Input: part model. Units: mm. Frame: model coordinates. A direction names the side the tool comes from. Give positions to 0.01 mm unless a question says otherwise; leave off trailing zeros. Order: outer loops, then holes, each group sorted by start corner. A loop starts at its lowest first (then second) coordinate and runs counter-clockwise, first axis right, second up.
```python
from build123d import *

# Parameters (mm, degrees)
F0_W     = 41.91
F0_H     = 2.54
F1_DEPTH = 15.24
F0_H_2   = 24.13
F2_DEPTH = 2.54


with BuildPart() as f1:
    # F0 (on Front) → F1 (new body)
    with BuildSketch(Plane.XZ):
        with Locations((20.955, 25.4)):
            Rectangle(F0_W, F0_H)
        Polygon((41.91, 24.13), (41.91, 0), (41.91, -2.54), (44.45, -2.54), (44.45, 26.67), (41.91, 26.67), align=None)
        with Locations((20.955, -1.27)):
            Rectangle(F0_W, F0_H)
    extrude(amount=F1_DEPTH)

    # F0 (on Front) → F2 (join)
    with BuildSketch(Plane.XZ):
        with Locations((20.955, 12.065)):
            Rectangle(F0_W, F0_H_2)
    extrude(amount=F2_DEPTH)


solid = f1.part
```
1) Reachability of faces 5 (the face through (21, -2.54, 12)), 6 (the face through (25, -15.24, -1)) from +Z, -Z, +X, -X, +Y, -Y: full face, straight path, thin tool, end or side. Return the list, or none.
2) Cut plane A-A (y = -8.5). Return the cut outline in (x, z), then the cut area to 3 significant figures.
3) Line query: probe 1 along Z at (x, y) = (41.5, -7.5); probe 2 along X at (y, z) = (-9, 16.5); probe 3 along Y at (x, z) = (27.5, 11). Output: solid intervals per line, ascending.
4) Cut plane B-B (x = 39). Return the cut outline in (y, z).
5) Pull-direction query (Z, two-part tool) for faces 1 (the face through (23, -8, 26.67)), 2 (the face through (41.91, -9, 12)), 3 (the face through (21, -9, 24.13)), 4 (the face through (44.45, -8, 12)); classes: pulls with the +Z half, pulls with the -Z half, needs draft (parallel to the pull), parting line crosses it, or undercut.
6) First-contact query: P1, Ø10, axis at x = 15, z = 13.5, coming from the -Y side; P2, Ø4, axis at y = -11, z = 17, coming from the -X side. Flat tips, straight axial feed; report the tip coordinate or a pass-through.
7) Cut plane C-C (z = 19.75). Return the cut outline in (x, y), then the cut area to 3 significant figures.
Geometry says:
1. face 5: -X, -Y
1. face 6: +Z, -Z, +X, -X, -Y
2. outline: (0, -2.54) - (44.45, -2.54) - (44.45, 26.67) - (0, 26.67) - (0, 24.13) - (41.91, 24.13) - (41.91, 0) - (0, 0) - close
2. area: 287 mm2
3. probe 1: z = -2.54 to 0, 24.13 to 26.67
3. probe 2: x = 41.91 to 44.45
3. probe 3: y = -2.54 to 0
4. outline: (-15.24, -2.54) - (0, -2.54) - (0, 26.67) - (-15.24, 26.67) - (-15.24, 24.13) - (-2.54, 24.13) - (-2.54, 0) - (-15.24, 0) - close
5. face 1: pulls with the +Z half
5. face 2: undercut
5. face 3: undercut
5. face 4: needs draft
6. P1: stops at y = -2.54
6. P2: stops at x = 41.91
7. outline: (0, -2.54) - (41.91, -2.54) - (41.91, -15.24) - (44.45, -15.24) - (44.45, 0) - (0, 0) - close
7. area: 145 mm2
